Design review of the part built by this model. Coordinates are the model's own, in mm. Face numbers are marked on the shaded views. Give positions to 0.01 mm unless a question says otherwise; leave off trailing zeros. Write each loop counter-clockwise with the first axis right and the second up, starting at its lowest first coordinate (ties: lowest second). Pieces come first, ordered by that corner, then holes. Notation, with made-up numbers: M 0,5.25 L 14,5.25 A29 ccw 14,39.25 Z; hole C 19.25,84.5 d9. An arc over 180 degrees is marked long. One line per item, written item: value. Start each with the question number.
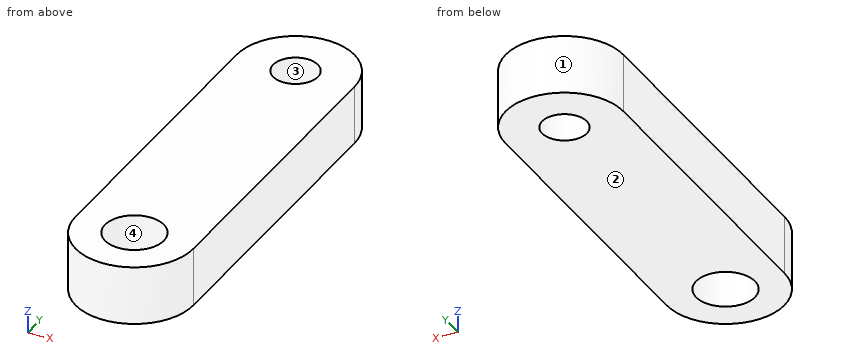
Autodesk Inventor part; units mm, degrees
ref_plane "YZ Plane" through (0, 0, 0) normal (1, 0, 0) x (0, 1, 0)
ref_plane "XZ Plane" through (0, 0, 0) normal (0, 1, 0) x (-1, 0, 0)
ref_plane "XY Plane" through (0, 0, 0) normal (0, 0, 1) x (1, 0, 0)
sketch "Sketch1" plane through (0, 0, 0) normal (0, 0, 1) x (1, 0, 0)
  line L0 (0, -16.6688) -> (0, 16.6688) construction
  line L1 (-6.35, -16.6688) -> (-6.35, 16.6688)
  line L2 (6.35, 16.6688) -> (6.35, -16.6687)
  arc A0 (-6.35, -16.6688) -> (6.35, -16.6687) centre (0, -16.6688) ccw
  arc A1 (6.35, 16.6688) -> (-6.35, 16.6688) centre (0, 16.6688) ccw
  circle A2 centre (0, 16.6688) radius 2.413
  circle A3 centre (0, -16.6688) radius 3.175
  point P0 (0, 0)
  dimension "d0" = 16.6687
  dimension "d1" = 4.826
  dimension "d2" = 6.35
  dimension "d3" = 6.35
extrude "Extrusion1" add sketch "Sketch1" along normal blind 6.35
properties part number "Dog Shifter Reverse Connector Plate" material "Aluminum 6061"
Q1. Take a section at B-B, the plane y = -15. Give the boundary of the cut face in (x, z), then the cut area to 3 significant figures.
Q2. Take a section at C-C, the plane z = 1.25. Give the boundary of the cut face in (x, y) (3 decimals).
Q3. Take a section at D-D, the plane x = 4.5. Give the boundary of the cut face in (y, z).
Q4. Take a section at A-A, the plane x = 0. Give the boundary of the cut face in (y, z), then the cut area to 3 significant figures.
Q5. The part is to be moulded in two halves that separate along Y. For the marked faces 1, 2, 3 and 4, say which applies: pulls with the +Y half, pulls with the -Y half, needs draft (parallel to the pull), parting line crosses it, or undercut.
Q6. Wall thickness on line 1 (Y direction, x = 0, z = 3.5); line 2 (Y direction, x = -1.25, z = 2.75); line 3 (X direction, y = -16, z = 6): over which ranges is each line inside the solid? List them lowest first. Write a range as from..to.
Q7. For P1, Ø1, axis at x = -5, z = 2.5, coming from the +Y side, flat-tipped, find the tip position at first contact; note if it passes through.
Results list:
1. outline: M -6.35,0 L -2.7,0 L -2.7,6.35 L -6.35,6.35 Z; M 2.7,0 L 6.35,0 L 6.35,6.35 L 2.7,6.35 Z
1. area: 46.3 mm^2
2. outline: M -6.35,-16.669 A6.35 ccw 6.35,-16.669 L 6.35,16.669 A6.35 ccw -6.35,16.669 Z; hole C 0,-16.669 d6.35; hole C 0,16.669 d4.826
3. outline: M -21.15,0 L 21.15,0 L 21.15,6.35 L -21.15,6.35 Z
4. outline: M -23.02,0 L -19.84,0 L -19.84,6.35 L -23.02,6.35 Z; M -13.49,0 L 14.26,0 L 14.26,6.35 L -13.49,6.35 Z; M 19.08,0 L 23.02,0 L 23.02,6.35 L 19.08,6.35 Z
4. area: 221 mm^2
5. face 1: pulls with the +Y half
5. face 2: needs draft
5. face 3: undercut
5. face 4: undercut
6. line 1: y = -23.02..-19.84, -13.49..14.26, 19.08..23.02
6. line 2: y = -22.89..-19.59, -13.75..14.6, 18.73..22.89
6. line 3: x = -6.35..-3.1, 3.1..6.35
7. P1: stops at y = 21.15
